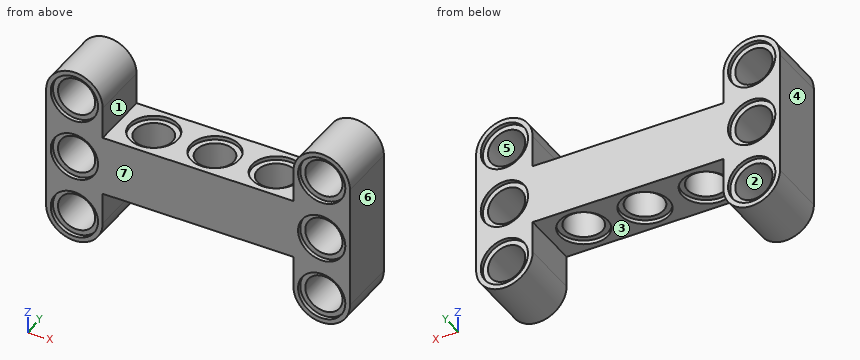
from build123d import *

# Parameters (mm, degrees)
SKETCH1_R           = 2.4
BOSS_EXTRUDE2_DEPTH = 7.7
SKETCH2_R           = 3.05
SKETCH2_R_2         = 2.4
CUT_EXTRUDE3_DEPTH  = 0.5
SKETCH3_R           = 2.4
CUT_EXTRUDE4_DEPTH  = 16.45
SKETCH4_R           = 3.1
SKETCH4_R_2         = 2.4
CUT_EXTRUDE6_DEPTH  = 0.5


with BuildPart() as part:
    # Sketch1 → Boss-Extrude2 (new body)
    with BuildSketch(Plane(origin=(0, 0, 0), x_dir=(1, 0, 0), z_dir=(0, 1, 0))):
        with BuildLine():
            Line((19.6, 4.1), (19.6, -11.8))
            ThreePointArc((19.6, -11.8), (15.95, -15.45), (12.3, -11.8))
            Line((12.3, -11.8), (12.3, -7.7))
            Line((12.3, -7.7), (-12.3, -7.7))
            Line((-12.3, -7.7), (-12.3, -11.8))
            ThreePointArc((-12.3, -11.8), (-15.95, -15.45), (-19.6, -11.8))
            Line((-19.6, -11.8), (-19.6, 4.1))
            ThreePointArc((-19.6, 4.1), (-15.95, 7.75), (-12.3, 4.1))
            Line((-12.3, 4.1), (-12.3, 0))
            Line((-12.3, 0), (12.3, 0))
            Line((12.3, 0), (12.3, 4.1))
            ThreePointArc((12.3, 4.1), (15.95, 7.75), (19.6, 4.1))
        make_face()
        with Locations((15.95, 4.1)):
            Circle(SKETCH1_R, mode=Mode.SUBTRACT)
        with Locations((15.95, -3.85)):
            Circle(SKETCH1_R, mode=Mode.SUBTRACT)
        with Locations((15.95, -11.8)):
            Circle(SKETCH1_R, mode=Mode.SUBTRACT)
        with Locations((-15.95, -11.8)):
            Circle(SKETCH1_R, mode=Mode.SUBTRACT)
        with Locations((-15.95, -3.85)):
            Circle(SKETCH1_R, mode=Mode.SUBTRACT)
        with Locations((-15.95, 4.1)):
            Circle(SKETCH1_R, mode=Mode.SUBTRACT)
    extrude(amount=BOSS_EXTRUDE2_DEPTH)

    # Sketch2 → Cut-Extrude3 (cut)
    with BuildSketch(Plane(origin=(0, 7.7, 0), x_dir=(1, 0, 0), z_dir=(0, 1, 0))):
        with Locations((-15.95, 4.1)):
            Circle(SKETCH2_R)
        with Locations((-15.95, 4.1)):
            Circle(SKETCH2_R_2, mode=Mode.SUBTRACT)
        with Locations((-15.95, -3.85)):
            Circle(SKETCH2_R)
        with Locations((-15.95, -3.85)):
            Circle(SKETCH2_R_2, mode=Mode.SUBTRACT)
        with Locations((-15.95, -11.8)):
            Circle(SKETCH2_R)
        with Locations((-15.95, -11.8)):
            Circle(SKETCH2_R_2, mode=Mode.SUBTRACT)
        with Locations((15.95, -3.85)):
            Circle(SKETCH2_R)
        with Locations((15.95, -3.85)):
            Circle(SKETCH2_R_2, mode=Mode.SUBTRACT)
        with Locations((15.95, 4.1)):
            Circle(SKETCH2_R)
        with Locations((15.95, 4.1)):
            Circle(SKETCH2_R_2, mode=Mode.SUBTRACT)
        with Locations((15.95, -11.8)):
            Circle(SKETCH2_R)
        with Locations((15.95, -11.8)):
            Circle(SKETCH2_R_2, mode=Mode.SUBTRACT)
    cut_extrude3 = extrude(amount=-CUT_EXTRUDE3_DEPTH, mode=Mode.SUBTRACT)

    # Sketch3 → Cut-Extrude4 (cut, through all)
    with BuildSketch(Plane(origin=(0, 0, 0), x_dir=(-1, 0, 0), z_dir=(0, 0, -1))):
        with Locations((7.9, 3.85)):
            Circle(SKETCH3_R)
        with Locations((0, 3.85)):
            Circle(SKETCH3_R)
        with Locations((-7.9, 3.85)):
            Circle(SKETCH3_R)
    extrude(amount=-CUT_EXTRUDE4_DEPTH, mode=Mode.SUBTRACT)

    # Sketch4 → Cut-Extrude6 (cut)
    with BuildSketch(Plane(origin=(0, 0, 0), x_dir=(-1, 0, 0), z_dir=(0, 0, -1))):
        with Locations((-7.9, 3.85)):
            Circle(SKETCH4_R)
        with Locations((-7.9, 3.85)):
            Circle(SKETCH4_R_2, mode=Mode.SUBTRACT)
        with Locations((0, 3.85)):
            Circle(SKETCH4_R)
        with Locations((0, 3.85)):
            Circle(SKETCH4_R_2, mode=Mode.SUBTRACT)
        with Locations((7.9, 3.85)):
            Circle(SKETCH4_R)
        with Locations((7.9, 3.85)):
            Circle(SKETCH4_R_2, mode=Mode.SUBTRACT)
    cut_extrude6 = extrude(amount=-CUT_EXTRUDE6_DEPTH, mode=Mode.SUBTRACT)

    # Mirror1: Cut-Extrude6 across plane
    add(cut_extrude6.mirror(Plane(origin=(0, 0, 3.85), x_dir=(1, 0, 0), z_dir=(0, 0, -1))), mode=Mode.SUBTRACT)

    # Mirror2: Cut-Extrude3 across plane
    add(cut_extrude3.mirror(Plane.ZX.offset(3.85)), mode=Mode.SUBTRACT)


solid = part.part
CAD build for the part. Positions are in the model's coordinates, mm. Face numbers are marked on the shaded views. A direction names the side the tool comes from. Give positions to 0.01 mm unless a question says otherwise; leave off trailing zeros. Order: outer loops, then holes, each group sorted by start corner. A loop starts at its lowest first (then second) coordinate and runs counter-clockwise, first axis right, second up. Notation, with made-up numbers: (42, 6.25) - (71, 6.25) arc R18 cw to (71, 32.25) - close; hole circle Ø8 at (33, -12). An arc over 180 degrees is marked (long way). Write each question's results on one line, items separated by ' | '.
1. Pin check, flat tips, straight feed: pin 1 (5 mm diameter, centred on x = 16, z = 12, fed in from +Y); pin 2 (5 mm diameter, centred on x = 15.95, z = -4.1, fed in from -Y); pin 3 (3 mm diameter, centred on x = 9, y = 4, fed in from +Z). Stop position of each tip, or through.
Calculated:
pin 1: stops at y = 7.2 | pin 2: stops at y = 0.5 | pin 3: stops at z = 7.2
2. Saw through at B-B on x = 7.9. List the corners of the cut face in (y, z), and give its area (3 significant figures).
Calculated:
outline: (0, 0) - (0.75, 0) - (0.75, 0.5) - (1.45, 0.5) - (1.45, 7.2) - (0.75, 7.2) - (0.75, 7.7) - (0, 7.7) - close; (6.25, 0.5) - (6.95, 0.5) - (6.95, 0) - (7.7, 0) - (7.7, 7.7) - (6.95, 7.7) - (6.95, 7.2) - (6.25, 7.2) - close | area: 20.9 mm2
3. Probe L1, parallel to Z at x = -15.95, y = 0.3; L2, parallel to X at y = 2.5, z = -4.25; L3, parallel to Z at x = 16, y = 6. List the from-to ranges inside material, lowest first. Write a range as from..to.
Calculated:
L1: z = -7.75..-7.15, -1.05..0.8, 6.9..8.75, 14.85..15.45 | L2: x = -19.6..-18.35, -13.55..-12.3, 12.3..13.55, 18.35..19.6 | L3: z = -7.75..-6.5, -1.7..1.45, 6.25..9.4, 14.2..15.45
4. Saw through at A-A on z = 3.85. Count the separate pieces of the cut face and the enclosed holes in it, and give its area (3 significant figures).
Calculated:
separate pieces: 3 | enclosed holes: 3 | area: 171 mm2
5. 3-axis set-ups, long thin cutter, end or side, ignore diameter. For the marked faces 1, 2 and 3: which of +Z, -Z, +X, -X, +Y, -Y reach the whole face in a straight line?
Calculated:
face 1: +Z, +Y, -Y | face 2: +Y, -Y | face 3: -Z, +Y, -Y
6. Pull direction X, two halves, no side cores. Call the marked faces 4, 5, 6 and 7: released by +X, released by -X, zero draft, split by the parting line, or undercut.
Calculated:
face 4: released by -X | face 5: undercut | face 6: released by +X | face 7: zero draft
